Check sheet for the drawn part. Datum: minimum x, y, z corner. Units: mm. A direction names the side the tool comes from. Give positions to 0.01 mm unless a question says otherwise; leave off trailing zeros. Loops run counter-clockwise (first coordinate to the right, second up) from the corner with the lowest first, then second, coordinate; pieces in that order, holes last.
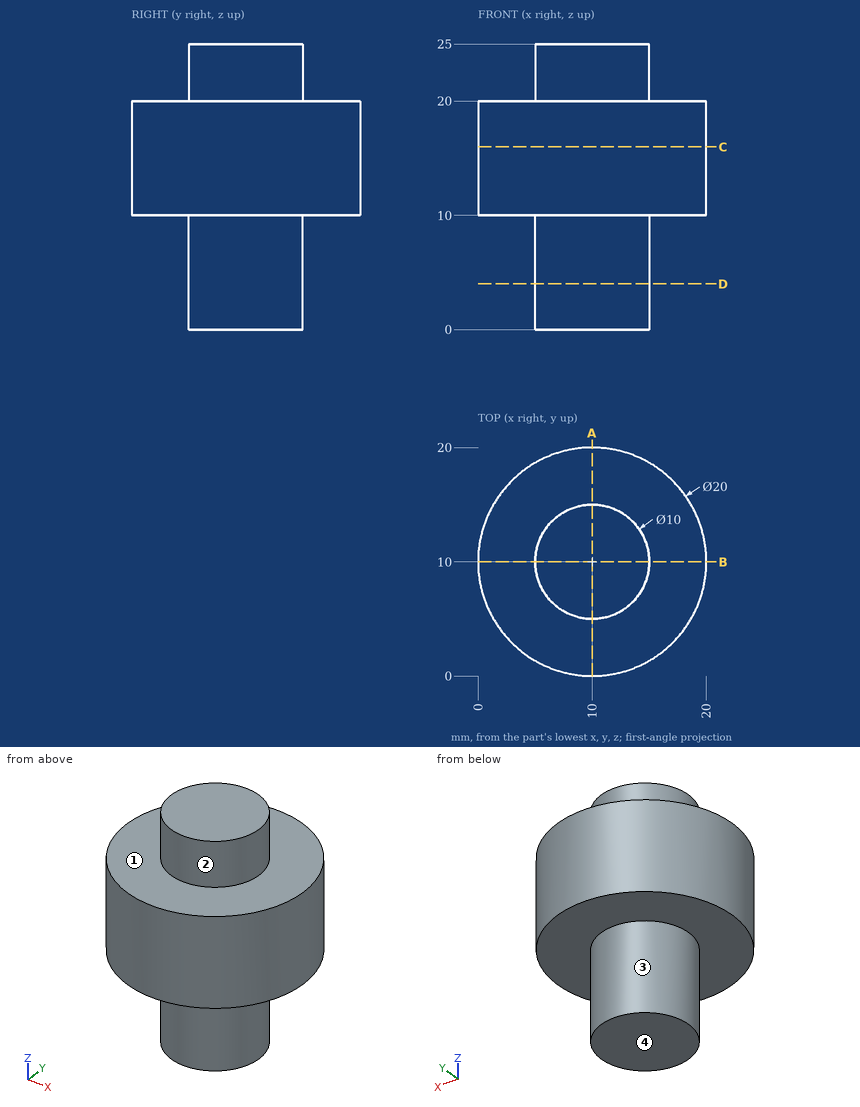
1) Sectioned sample at A-A on x = 10. Enter the section's corners in (y, z).
2) Tool access check on the marked faces 3 and 4. Record the directions out of +Z, -Z, +X, -X, +Y, -Y that give a thin tool (end or side, any length) a straight path to the whole face; none if there is none.
3) Mould release check, pull along Y, two halves, no side actions. Record for the marked faces 1 and 2: +Y half, -Y half, draft (parallel to the pull), parting line (faces both ways), or undercut.
4) Scan lines: line 1 along Z through (x, y) = (7.25, 16.5); line 2 along Y through (x, z) = (12.75, 22.75); line 3 along Y through (x, z) = (7.5, 12). Record each from-to range of solid material in increasing order.
5) Depth check by flat-ended pin: P1, Ø10, axis at x = 10, z = 20.5, coming from the -Y side; P2, Ø1, axis at x = 16, y = 14.5, coming from the -Z side; P3, Ø2, axis at x = 7, z = 20.5, coming from the -Y side; P4, Ø1.5, axis at y = 2, z = 11.5, coming from the +X side. Enter the tip coordinate at first touch or a pass-through.
6) Sectioned sample at D-D on z = 4. Enter the section's corners in (x, y).
7) Sectioned sample at C-C on z = 16. Enter the section's corners in (x, y).
Determined:
1. outline: (0, 10) - (5, 10) - (5, 0) - (15, 0) - (15, 10) - (20, 10) - (20, 20) - (15, 20) - (15, 25) - (5, 25) - (5, 20) - (0, 20) - close
2. face 3: -Z
2. face 4: -Z, +X, -X, +Y, -Y
3. face 1: draft
3. face 2: parting line
4. line 1: z = 10 to 20
4. line 2: y = 5.82 to 14.18
4. line 3: y = 0.32 to 19.68
5. P1: stops at y = 0
5. P2: stops at z = 10
5. P3: stops at y = 0.23
5. P4: stops at x = 16.89
6. outline: circle Ø10 at (10, 10)
7. outline: circle Ø20 at (10, 10)
